```python
from build123d import *

# Parameters (mm, degrees)
SKETCH1_W                 = 36
SKETCH1_H                 = 36
BOSS_EXTRUDE1_DEPTH       = 15
SKETCH2_R                 = 10
CUT_EXTRUDE1_DEPTH        = 4
SKETCH4_R                 = 10
CUT_EXTRUDE2_DEPTH        = 4
M8X1_0_TAPPED_HOLE1_D     = 7
M8X1_0_TAPPED_HOLE1_DEPTH = 15
M8X1_0_TAPPED_HOLE1_TIP   = 2.103012167
M8X1_0_TAPPED_HOLE2_D     = 7
M8X1_0_TAPPED_HOLE2_DEPTH = 15
M8X1_0_TAPPED_HOLE2_TIP   = 2.103012167
FILLET1_R                 = 10
M4X0_7_TAPPED_HOLE1_D     = 3.3
M4X0_7_TAPPED_HOLE1_DEPTH = 10.1
M4X0_7_TAPPED_HOLE1_TIP   = 0.991420021
CUT_EXTRUDE3_DEPTH        = 60.093146983
FILLET2_R                 = 1


with BuildPart() as part:
    # Sketch1 → Boss-Extrude1 (new, symmetric)
    with BuildSketch(Plane.XY):
        with Locations((-18, -18)):
            Rectangle(SKETCH1_W, SKETCH1_H)
    extrude(amount=BOSS_EXTRUDE1_DEPTH, both=True)

    # Sketch2 → Cut-Extrude1 (cut)
    with BuildSketch(Plane.XZ.offset(36)):
        with Locations((-19.294, 0)):
            Circle(SKETCH2_R)
    extrude(amount=-CUT_EXTRUDE1_DEPTH, mode=Mode.SUBTRACT)

    # Sketch4 → Cut-Extrude2 (cut)
    with BuildSketch(Plane.ZY.offset(36)):
        with Locations(Location((0, -19.294, 0), (0, 0, 270))):
            Circle(SKETCH4_R)
    extrude(amount=-CUT_EXTRUDE2_DEPTH, mode=Mode.SUBTRACT)

    # M8x1.0 Tapped Hole1
    with Locations(Plane.ZY.offset(32)):
        with Locations((0, -19.294)):
            Hole(M8X1_0_TAPPED_HOLE1_D / 2, depth=M8X1_0_TAPPED_HOLE1_DEPTH)
            with Locations((0, 0, -(M8X1_0_TAPPED_HOLE1_DEPTH + M8X1_0_TAPPED_HOLE1_TIP / 2))):  # 118° drill point
                Cone(0, M8X1_0_TAPPED_HOLE1_D / 2, M8X1_0_TAPPED_HOLE1_TIP, mode=Mode.SUBTRACT)

    # M8x1.0 Tapped Hole2
    with Locations(Plane.XZ.offset(32)):
        with Locations((-19.294, 0)):
            Hole(M8X1_0_TAPPED_HOLE2_D / 2, depth=M8X1_0_TAPPED_HOLE2_DEPTH)
            with Locations((0, 0, -(M8X1_0_TAPPED_HOLE2_DEPTH + M8X1_0_TAPPED_HOLE2_TIP / 2))):  # 118° drill point
                Cone(0, M8X1_0_TAPPED_HOLE2_D / 2, M8X1_0_TAPPED_HOLE2_TIP, mode=Mode.SUBTRACT)

    # Fillet1
    # the kernel refuses this fillet: 10 mm, written as the material it takes off along each edge
    with BuildSketch(Plane(origin=(0, -36, 40), x_dir=(0, 1, 0), z_dir=(0, 0, -1)), Plane(origin=(-36, 0, -40), x_dir=(1, 0, 0), z_dir=(0, 0, 1))) as fillet1_piece_1:
        with BuildLine():
            CenterArc((FILLET1_R, -FILLET1_R), FILLET1_R, 90, 90)
            Line((0, -FILLET1_R), (0, 0))
            Line((0, 0), (FILLET1_R, 0))
        make_face()
    extrude(amount=80, mode=Mode.SUBTRACT)
    with BuildSketch(Plane(origin=(-36, -36, -40), x_dir=(1, 0, 0), z_dir=(0, 0, 1))) as fillet1_piece_2:
        with BuildLine():
            CenterArc((FILLET1_R, FILLET1_R), FILLET1_R, 180, 90)
            Line((0, FILLET1_R), (0, 0))
            Line((0, 0), (FILLET1_R, 0))
        make_face()
    extrude(amount=80, mode=Mode.SUBTRACT)

    # M4x0.7 Tapped Hole1
    with Locations(Plane(origin=(0, 0, -15), x_dir=(-1, 0, 0), z_dir=(0, 0, -1))):
        with Locations((29.900601718, -29.900601718), (4.805112606, -23.176285677), (23.176285677, -4.805112606)):
            Hole(M4X0_7_TAPPED_HOLE1_D / 2, depth=M4X0_7_TAPPED_HOLE1_DEPTH)
            with Locations((0, 0, -(M4X0_7_TAPPED_HOLE1_DEPTH + M4X0_7_TAPPED_HOLE1_TIP / 2))):  # 118° drill point
                Cone(0, M4X0_7_TAPPED_HOLE1_D / 2, M4X0_7_TAPPED_HOLE1_TIP, mode=Mode.SUBTRACT)

    # Sketch12 → Cut-Extrude3 (cut, through all)
    with BuildSketch(Plane(origin=(0, 0, -15), x_dir=(-1, 0, 0), z_dir=(0, 0, -1))):
        Polygon((0, -12.425049096), (12.425049096, 0), (0, 0), align=None)
    extrude(amount=-CUT_EXTRUDE3_DEPTH, mode=Mode.SUBTRACT)

    # Fillet2
    fillet2_edges = [part.edges().sort_by_distance(p)[0] for p in [
        (0, -12.425049096, 0),
        (-6.212524548, -6.212524548, 15),
        (-12.425049096, 0, 0),
        (-6.212524548, -6.212524548, -15),
        (-36, -18, -15),
        (-36, -18, 15),
        (0, -19.212524548, -15),
        (-18, -36, -15),
        (-33.071067812, -33.071067812, -15),
        (-2.928932188, -33.071067812, -15),
        (-33.071067812, -2.928932188, -15),
        (0, -19.212524548, 15),
        (-18, -36, 15),
        (-33.071067812, -33.071067812, 15),
        (-2.928932188, -33.071067812, 15),
        (-33.071067812, -2.928932188, 15),
        (-19.212524548, 0, -15),
        (-19.212524548, 0, 15),
    ]]
    fillet(fillet2_edges, radius=FILLET2_R)


solid = part.part
```
The listing builds one solid part. Answer for the finished solid, in the listing's coordinates (mm). A direction names the side the tool comes from. Round coordinates to 2 decimals unless told otherwise and drop trailing zeros. Loops run counter-clockwise (first coordinate to the right, second up) from the corner with the lowest first, then second, coordinate; pieces in that order, holes last. Notation, with made-up numbers: (43.25, 69) - (62.25, 69) arc R17 cw to (62.25, 74) - close; hole circle Ø10 at (-8.75, 4.25). An arc over 180 degrees is marked (long way). Return JSON: item names as keys, results as strings. Group by question number.
1. Each of these flat-tipped pins is pushed along its axis until it touches: P1, Ø1, axis at x = -6, z = -7.5, coming from the +Y side; P2, Ø8, axis at x = -19.294, z = 0, coming from the -Y side; P3, Ø1.5, axis at x = -27, z = 11, coming from the -Y side. Where does it stop, or does it pass through?
2. The mould has two halves that part along X. Classify faces 1 (the cylindrical face through (-35.715, -17.888, 14.699)), 2 (the conical face through (-22.89, -4.79, -4.08)), 3 (the conical face through (-18.714, -15.262, 0.183)), 4 (the cylindrical face through (-6.5, -6.33, -14.7)): pulls with the +X half, pulls with the -X half, needs draft (parallel to the pull), parting line crosses it, or undercut.
3. The part is cut by section A-A on z = -6.5. Determine the outline of the cut face in (x, y), then the cut area to 3 significant figures.
4. Consider probe 1 along Z at (x, y) = (-25, -18); probe 2 along Y at (x, z) = (-32.5, 4); probe 3 along Y at (x, z) = (-20, 9.5). Determine where each line is inside the solid, lowest interval first.
5. The part is cut by section B-B on z = -12. Determine the outline of the cut face in (x, y), then the cut area to 3 significant figures.
6. Which of the six approach directions +Z, -Z, +X, -X, +Y, -Y give full straight-line access (tool end or side, diameter ignored) to faces 5 (the cylindrical face through (-0.301, -19.512, -14.715)), 6 (the cylindrical face through (-5.163, -24.787, -9.879)), 7 (the cylindrical face through (-34.028, -9.304, 0.44))?
Resolved:
{
 "1": {"P1": "stops at y = -5.93", "P2": "stops at y = -32", "P3": "stops at y = -36"},
 "2": {"face 1": "pulls with the -X half", "face 2": "undercut", "face 3": "undercut", "face 4": "pulls with the +X half"},
 "3": {"outline": "(-36, -11.69) - (-32, -11.69) - (-32, -26.89) - (-35.96, -26.89) arc R10 ccw to (-26.89, -35.96) - (-26.89, -32) - (-11.69, -32) - (-11.69, -36) - (-10, -36) arc R10 ccw to (0, -26) - (0, -12.84) arc R1 ccw to (-0.29, -12.13) - (-12.13, -0.29) arc R1 ccw to (-12.84, 0) - (-26, 0) arc R10 ccw to (-36, -10) - close; hole circle Ø3.3 at (-29.9, -29.9); hole circle Ø3.3 at (-23.18, -4.81); hole circle Ø3.3 at (-4.81, -23.18)", "area": "1,010 mm²"},
 "4": {"probe 1": "z = -15 to -3.25, 3.25 to 15", "probe 2": "y = -33.6 to -28.46, -10.13 to -2.4", "probe 3": "y = -32 to 0"},
 "5": {"outline": "(-36, -26) arc R10 ccw to (-26, -36) - (-10, -36) arc R10 ccw to (0, -26) - (0, -12.84) arc R1 ccw to (-0.29, -12.13) - (-12.13, -0.29) arc R1 ccw to (-12.84, 0) - (-26, 0) arc R10 ccw to (-36, -10) - close; hole circle Ø3.3 at (-29.9, -29.9); hole circle Ø3.3 at (-23.18, -4.81); hole circle Ø3.3 at (-4.81, -23.18)", "area": "1,130 mm²"},
 "6": {"face 5": "-Z, +X, +Y, -Y", "face 6": "-Z", "face 7": "-X"}
}
